```python
from build123d import *

# Parameters (mm, degrees)
EXTRUDE_1_DEPTH     = 8.8
EXTRUDE_2_DEPTH     = 1.5
SKETCH_3_R          = 0.5
SKETCH_3_R_2        = 0.502704905
CUT_EXTRUDE_1_DEPTH = 0.1


with BuildPart() as part:
    # 草圖1 → 填料-伸長1 (new body)
    with BuildSketch(Plane.XY):
        with BuildLine():
            Line((-25, -52.25), (25, -52.25))
            ThreePointArc((25, -52.25), (32.071067812, -49.321067812), (35, -42.25))
            Line((35, -42.25), (35, 42.25))
            ThreePointArc((35, 42.25), (32.071067812, 49.321067812), (25, 52.25))
            Line((25, 52.25), (-25, 52.25))
            ThreePointArc((-25, 52.25), (-32.071067812, 49.321067812), (-35, 42.25))
            Line((-35, 42.25), (-35, -42.25))
            ThreePointArc((-35, -42.25), (-32.071067812, -49.321067812), (-25, -52.25))
        make_face()
    extrude(amount=EXTRUDE_1_DEPTH)

    # 草圖2 → 填料-伸長2 (add)
    with BuildSketch(Plane(origin=(0, 52.25, 0), x_dir=(1, 0, 0), z_dir=(0, 1, 0))):
        with BuildLine():
            Line((-16.5, -5.9), (-7.5, -5.9))
            ThreePointArc((-7.5, -5.9), (-7.146446609, -5.753553391), (-7, -5.4))
            Line((-7, -5.4), (-7, -3.4))
            ThreePointArc((-7, -3.4), (-7.146446609, -3.046446609), (-7.5, -2.9))
            Line((-7.5, -2.9), (-16.5, -2.9))
            ThreePointArc((-16.5, -2.9), (-16.853553391, -3.046446609), (-17, -3.4))
            Line((-17, -3.4), (-17, -5.4))
            ThreePointArc((-17, -5.4), (-16.853553391, -5.753553391), (-16.5, -5.9))
        make_face()
        with BuildLine():
            Line((7.5, -5.9), (16.5, -5.9))
            ThreePointArc((16.5, -5.9), (16.853553391, -5.753553391), (17, -5.4))
            Line((17, -5.4), (17, -3.4))
            ThreePointArc((17, -3.4), (16.853553391, -3.046446609), (16.5, -2.9))
            Line((16.5, -2.9), (7.5, -2.9))
            ThreePointArc((7.5, -2.9), (7.146446609, -3.046446609), (7, -3.4))
            Line((7, -3.4), (7, -5.4))
            ThreePointArc((7, -5.4), (7.146446609, -5.753553391), (7.5, -5.9))
        make_face()
    extrude(amount=EXTRUDE_2_DEPTH)

    # 草圖3 → 除料-伸長1 (cut)
    with BuildSketch(Plane(origin=(0, 0, 0), x_dir=(-1, 0, 0), z_dir=(0, 0, -1))):
        with Locations((0, 48.370695597)):
            Circle(SKETCH_3_R)
        with Locations((-2, 48.370695597)):
            Circle(SKETCH_3_R_2)
        with Locations((4, 48.370695597)):
            Circle(SKETCH_3_R)
        with Locations((2, 48.370695597)):
            Circle(SKETCH_3_R_2)
        with Locations((-4, 48.370695597)):
            Circle(SKETCH_3_R_2)
    extrude(amount=-CUT_EXTRUDE_1_DEPTH, mode=Mode.SUBTRACT)


solid = part.part
```
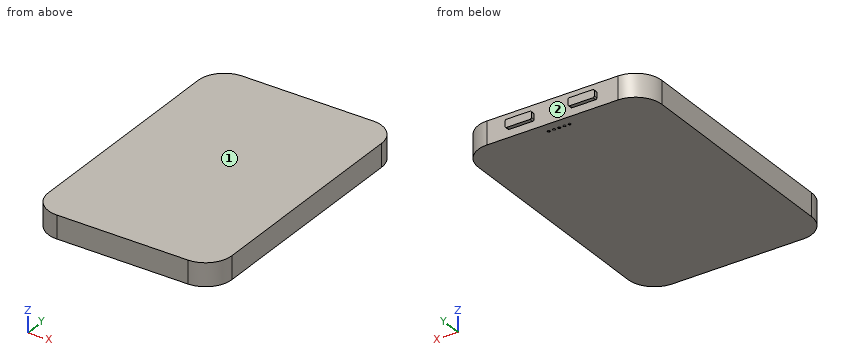
Could you check a few things on this model? Use its own coordinates, in mm. Face numbers are marked on the shaded views. A direction names the side the tool comes from. Give positions to 0.01 mm unless a question says otherwise; leave off trailing zeros. One line per item, written item: value. Start each with the question number.
Item 1: Please list where these lines run through material, in increasing order: line 1 (Y direction, x = -2, z = 0.05); line 2 (Y direction, x = -20.5, z = 3.5); line 3 (Y direction, x = 30, z = 3). Write a range as from..to.
Item 2: I'm going to push flat-ended pins straight in: pin 1 (0.5 mm diameter, centred on x = 4, y = 48.5, fed in from -Z); pin 2 (0.8 mm diameter, centred on x = -12, y = 53, fed in from +Z); pin 3 (5 mm diameter, centred on x = 2, z = 4, fed in from +Y). Where does each tip first touch, or does it pass through?
Item 3: Which directions (+Z, -Z, +X, -X, +Y, -Y) give clear straight access to the entire face, cutting with the end or side of a thin tool? Please do the marked faces 1 and 2.
Geometry says:
1. line 1: -52.25..47.87, 48.87..52.25
1. line 2: -52.25..52.25
1. line 3: -50.91..50.91
2. pin 1: z = 0.1
2. pin 2: z = 5.9
2. pin 3: y = 52.25
3. face 1: +Z, +X, -X, +Y, -Y
3. face 2: +Y
